from build123d import *

# Parameters (mm, degrees)
F1_DEPTH = 6.35
F2_R     = 3.175
F3_DEPTH = 8.89


with BuildPart() as f1:
    # F0 (on Front) → F1 (new body)
    with BuildSketch(Plane.XZ):
        with BuildLine():
            ThreePointArc((2.2450640303, 2.2450640303), (2.9333175157, 1.2150198978), (3.175, 0))
            ThreePointArc((3.175, 0), (1.2150198978, -2.9333175157), (-2.2450640303, -2.2450640303))
            Line((-2.2450640303, -2.2450640303), (-6.7351920908, -6.7351920908))
            Line((-6.7351920908, -6.7351920908), (42.6051664613, -56.0755506429))
            ThreePointArc((42.6051664613, -56.0755506429), (47.0952942961, -56.0755499657), (47.0952940704, -51.5854221309))
            Line((47.0952940704, -51.5854221309), (39.0388281543, -43.5289562148))
            ThreePointArc((39.0388281543, -43.5289562148), (38.6295458387, -43.0784169906), (38.2652810646, -42.5907605738))
            Line((38.2652810646, -42.5907605738), (10.6113248497, -1.6098451326))
            ThreePointArc((10.6113248497, -1.6098451326), (9.8026513109, 0.0849170206), (9.525, 1.9420872869))
            Line((9.525, 1.9420872869), (9.525, 171.45))
            ThreePointArc((9.525, 171.45), (7.6651280605, 175.9401280605), (3.175, 177.8))
            Line((3.175, 177.8), (-3.175, 177.8))
            ThreePointArc((-3.175, 177.8), (-7.6651280605, 175.9401280605), (-9.525, 171.45))
            Line((-9.525, 171.45), (-9.525, 0))
            ThreePointArc((-9.525, 0), (-3.6450596933, 8.7999525472), (6.7351920908, 6.7351920908))
            Line((6.7351920908, 6.7351920908), (2.2450640303, 2.2450640303))
        make_face()
        with BuildLine():
            ThreePointArc((-2.2450640303, -2.2450640303), (-2.2450640303, 2.2450640303), (2.2450640303, 2.2450640303))
            Line((2.2450640303, 2.2450640303), (6.7351920908, 6.7351920908))
            ThreePointArc((6.7351920908, 6.7351920908), (-3.6450596933, 8.7999525472), (-9.525, 0))
            ThreePointArc((-9.525, 0), (-8.7999525472, -3.6450596933), (-6.7351920908, -6.7351920908))
            Line((-6.7351920908, -6.7351920908), (-2.2450640303, -2.2450640303))
        make_face()
    extrude(amount=F1_DEPTH)

    # F2 (on face) → F3 (join)
    with BuildSketch(Plane.XZ.offset(6.35)):
        with Locations((44.8502300401, -53.8304861612)):
            Circle(F2_R)
    extrude(amount=F3_DEPTH)


solid = f1.part
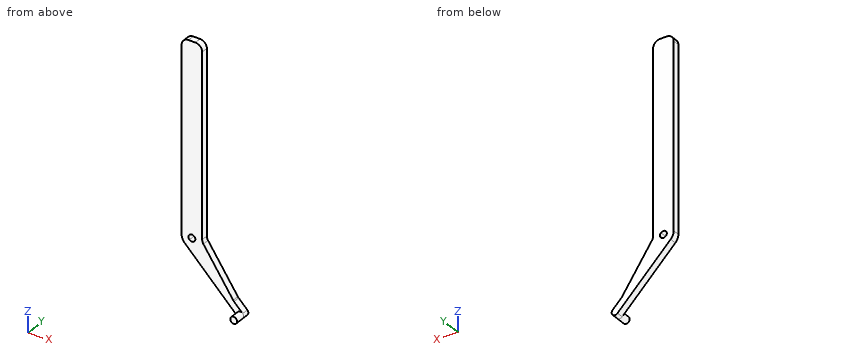
Model file for the job. Use its own axes, mm. Round coordinates to 2 decimals unless told otherwise and drop trailing zeros. Loops run counter-clockwise (first coordinate to the right, second up) from the corner with the lowest first, then second, coordinate; pieces in that order, holes last. Notation, with made-up numbers: (37.5, -9) -> (95.5, -9) arc R25 ccw to (95.5, 6) -> close; hole circle Ø5 at (34, -4). An arc over 180 degrees is marked (long way). Answer as CSV lines item,"result". Start each with the question number.
1) Probe line 1 along Y through (x, z) = (25, -29); line 2 along X through (y, z) = (-1.5, 83) (3 decimals); line 3 along Z through (x, y) = (44.5, -1.5). List the from-to ranges inside material, lowest first.
2) Slice it at B-B (z = 157). List the corners of the cut face in (x, y) (3 decimals).
3) Pin check, flat tips, straight feed: P1, Ø1.9, axis at y = -2.5, z = 121, coming from the +X side (3 decimals); P2, Ø6, axis at x = 2, y = -2.5, coming from the -Z side; P3, Ø8, axis at x = -3.5, z = 65.5, coming from the +Y side; P4, Ø6, axis at x = 1, z = -8.5, coming from the -Y side. Stop position of each tip, or through.
4) Slice it at D-D (y = -11). List the corners of the cut face in (x, z) (3 decimals).
5) Slice it at A-A (x = 0). List the corners of the cut face in (y, z) (3 decimals).
6) Slice it at C-C (x = 20). List the corners of the cut face in (y, z).
Filled in:
1,line 1,"y = -6.35 to 0"
1,line 2,"x = -9.525 to 9.525"
1,line 3,"z = -56.99 to -48.99"
2,outline,"(-9.525, -6.35) -> (9.525, -6.35) -> (9.525, 0) -> (-9.525, 0) -> close"
3,P1,"stops at x = 9.525"
3,P2,"stops at z = -18.47"
3,P3,"stops at y = 0"
3,P4,"stops at y = -6.35"
4,outline,"circle Ø6.35 at (44.85, -53.83)"
5,outline,"(-6.35, -13.47) -> (0, -13.47) -> (0, -3.175) -> (-6.35, -3.175) -> close; (-6.35, 3.175) -> (0, 3.175) -> (0, 177.8) -> (-6.35, 177.8) -> close"
6,outline,"(-6.35, -33.47) -> (0, -33.47) -> (0, -15.52) -> (-6.35, -15.52) -> close"
